Could you check a few things on this model? Use its own coordinates, in mm. Face numbers are marked on the shaded views. A direction names the side the tool comes from. Give positions to 0.01 mm unless a question says otherwise; leave off trailing zeros. Order: outer loops, then holes, each group sorted by start corner. A loop starts at its lowest first (then second) coordinate and runs counter-clockwise, first axis right, second up.
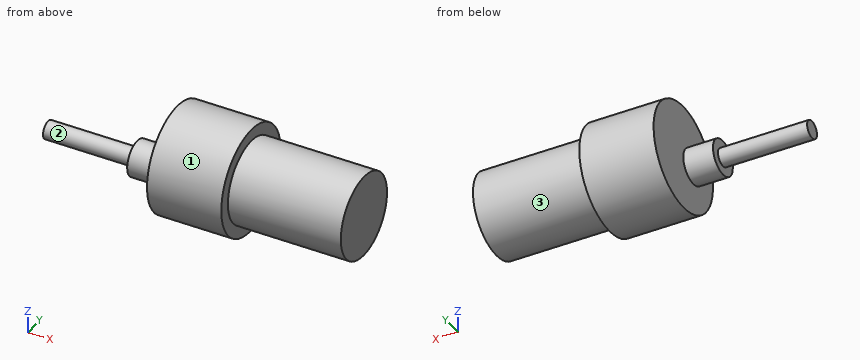
from build123d import *


with BuildPart() as part:
    # Sketch2 → Revolve2 (revolve)
    with BuildSketch(Plane.XY, mode=Mode.PRIVATE) as revolve2_sk:
        Polygon((46.393095281, 0), (46.393095281, 18), (71.393095281, 18), (71.393095281, 14), (109.393095281, 14), (109.393095281, 0), align=None)
    revolve(revolve2_sk.sketch.rotate(Axis((109.393095281, 0, 0), (-1, 0, 0)), 90), axis=Axis((109.393095281, 0, 0), (-1, 0, 0)))

    # Sketch13 → Revolve3 (revolve)
    with BuildSketch(Plane.XY, mode=Mode.PRIVATE) as revolve3_sk:
        Polygon((46.393095281, -6), (46.393095281, 0), (36.393095281, 0), (36.393095281, -3), (6.393095281, -3), (6.393095281, -6), align=None)
    revolve(revolve3_sk.sketch.rotate(Axis((46.393095281, -6, 0), (-1, 0, 0)), 90), axis=Axis((46.393095281, -6, 0), (-1, 0, 0)))


solid = part.part
Item 1: Imagine slicing it at C-C on x = 41. List the corners of the cut face in (y, z) for me.
Findings:
outline: circle Ø12 at (-6, 0)
Item 2: Please list where these lines run through material, in increasing order: line 1 along X through (y, z) = (-15.5, 9); line 2 along Y through (x, z) = (104, -3.5); line 3 along Y through (x, z) = (58, -2).
Findings:
line 1: x = 46.39 to 71.39
line 2: y = -13.56 to 13.56
line 3: y = -17.89 to 17.89
Item 3: Imagine slicing it at A-A on z = 0. List the corners of the cut face in (x, y) for me.
Findings:
outline: (6.39, -9) - (36.39, -9) - (36.39, -12) - (46.39, -12) - (46.39, -18) - (71.39, -18) - (71.39, -14) - (109.39, -14) - (109.39, 14) - (71.39, 14) - (71.39, 18) - (46.39, 18) - (46.39, 0) - (36.39, 0) - (36.39, -3) - (6.39, -3) - close
Item 4: Imagine slicing it at D-D on z = -11. List the corners of the cut face in (x, y) for me, then the cut area to 3 significant figures.
Findings:
outline: (46.39, -14.25) - (71.39, -14.25) - (71.39, -8.66) - (109.39, -8.66) - (109.39, 8.66) - (71.39, 8.66) - (71.39, 14.25) - (46.39, 14.25) - close
area: 1,370 mm2
Item 5: For the marked faces 1, 2 and 3, which set-ups out of +Z, -Z, +X, -X, +Y, -Y let a thin tool reach every point of the face, with its end or its side?
Findings:
face 1: +X, -X
face 2: -X
face 3: +X
Item 6: Imagine slicing it at B-B on y = -6. List the corners of the cut face in (x, z) for me, then the cut area to 3 significant figures.
Findings:
outline: (6.39, -3) - (36.39, -3) - (36.39, -6) - (46.39, -6) - (46.39, -16.97) - (71.39, -16.97) - (71.39, -12.65) - (109.39, -12.65) - (109.39, 12.65) - (71.39, 12.65) - (71.39, 16.97) - (46.39, 16.97) - (46.39, 6) - (36.39, 6) - (36.39, 3) - (6.39, 3) - close
area: 2,110 mm2
Item 7: For pin 1 (1 mm diameter, centred on x = 37.5, z = 5, fed in from +Y); pin 2 (10 mm diameter, centred on x = 35, z = -12, fed in from +Y); pin 3 (1 mm diameter, centred on x = 50, z = -5.5, fed in from +Y); pin 4 (12 mm diameter, centred on x = 22.5, z = 3.5, fed in from -Y), each with a flat end and sliding along its axis, tell me the tip position at first contact or that it passes through.
Findings:
pin 1: stops at y = -2.03
pin 2: passes through
pin 3: stops at y = 17.29
pin 4: stops at y = -9
